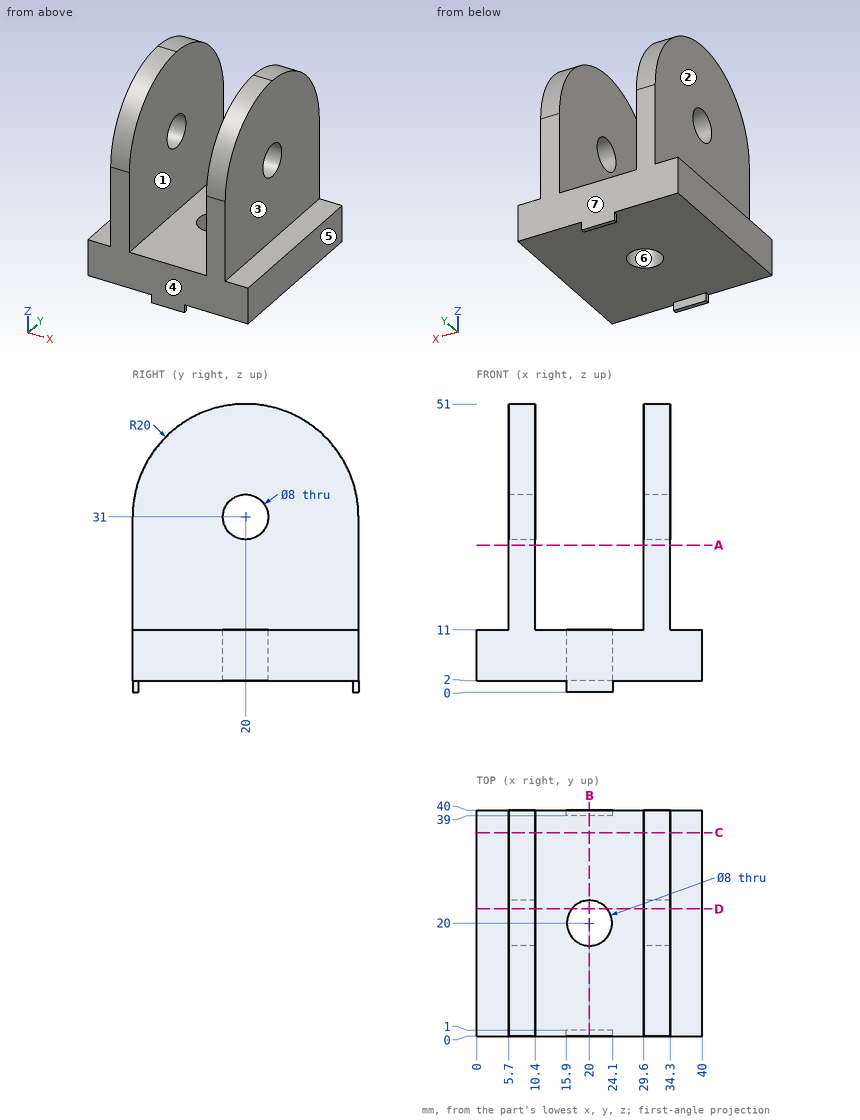
Job drawing, mm, ordinate dimensions from the low corner. One solid piece. A direction names the side the tool comes from. Round coordinates to 2 decimals unless told otherwise and drop trailing zeros. Loops run counter-clockwise (first coordinate to the right, second up) from the corner with the lowest first, then second, coordinate; pieces in that order, holes last.
(1) Drop flat-ended pins along their axis: pin 1 (4.5 mm diameter, centred on x = 38, y = 19.5, fed in from +Z); pin 2 (20 mm diameter, centred on x = 22, y = 13.5, fed in from -Z); pin 3 (0.5 mm diameter, centred on y = 39.5, z = 1, fed in from -X). Give the stop position or say it passes through.
(2) Cut at A-A (z = 26). Give the cut face in (x, y), plus the area to 3 significant figures.
(3) Cut at C-C (y = 36). Give the cut face in (x, z).
(4) Which spindle directions (+Z, -Z, +X, -X, +Y, -Y) get a long thin tool onto all of the face, cutting with end or side? Do the marked faces 1, 2 and 3. Say none if no direction does.
(5) Two-plate mould, pull along Y, no slides. Class the marked faces 4, 5, 6 and 7: +Y half, -Y half, draft (parallel to the pull), parting line (faces both ways), or undercut.
(6) Wall check: line 1 along Y through (x, z) = (7.6, 31); line 2 along X through (y, z) = (37.5, 32); line 3 along Z through (x, y) = (35, 32.5). Give the ranges that are in metal, low to high.
(7) Cut at B-B (x = 20). Give the cut face in (y, z).
(8) Cut at D-D (y = 22.5). Give the cut face in (x, z), plus the area to 3 significant figures.
Findings below:
1. pin 1: stops at z = 11
1. pin 2: stops at z = 2
1. pin 3: stops at x = 15.9
2. outline: (5.7, 0) - (10.4, 0) - (10.4, 40) - (5.7, 40) - close; (29.6, 0) - (34.3, 0) - (34.3, 40) - (29.6, 40) - close
2. area: 376 mm2
3. outline: (0, 2) - (40, 2) - (40, 11) - (34.3, 11) - (34.3, 43) - (29.6, 43) - (29.6, 11) - (10.4, 11) - (10.4, 43) - (5.7, 43) - (5.7, 11) - (0, 11) - close
4. face 1: +Z, +Y, -Y
4. face 2: +Z, -X, +Y, -Y
4. face 3: +Z, +X, +Y, -Y
5. face 4: -Y half
5. face 5: draft
5. face 6: undercut
5. face 7: +Y half
6. line 1: y = 0 to 16, 24 to 40
6. line 2: x = 5.7 to 10.4, 29.6 to 34.3
6. line 3: z = 2 to 11
7. outline: (0, 0) - (1, 0) - (1, 2) - (16, 2) - (16, 11) - (0, 11) - close; (24, 2) - (39, 2) - (39, 0) - (40, 0) - (40, 11) - (24, 11) - close
8. outline: (0, 2) - (16.88, 2) - (16.88, 11) - (10.4, 11) - (10.4, 27.88) - (5.7, 27.88) - (5.7, 11) - (0, 11) - close; (5.7, 34.12) - (10.4, 34.12) - (10.4, 50.84) - (5.7, 50.84) - close; (23.12, 2) - (40, 2) - (40, 11) - (34.3, 11) - (34.3, 27.88) - (29.6, 27.88) - (29.6, 11) - (23.12, 11) - close; (29.6, 34.12) - (34.3, 34.12) - (34.3, 50.84) - (29.6, 50.84) - close
8. area: 620 mm2
